The drawing under review shows one solid part. Ordinate dimensions are in mm from its lowest x, y, z. Coordinates: 2 decimals unless noted, no trailing zeros. Loops run counter-clockwise (first coordinate to the right, second up) from the corner with the lowest first, then second, coordinate; pieces in that order, holes last. Notation, with made-up numbers: M -22,16 L 33,16 A21 ccw 33,46 Z; hole C -12.5,37 d9. An arc over 180 degrees is marked long. Use one line per item in the form item = value.
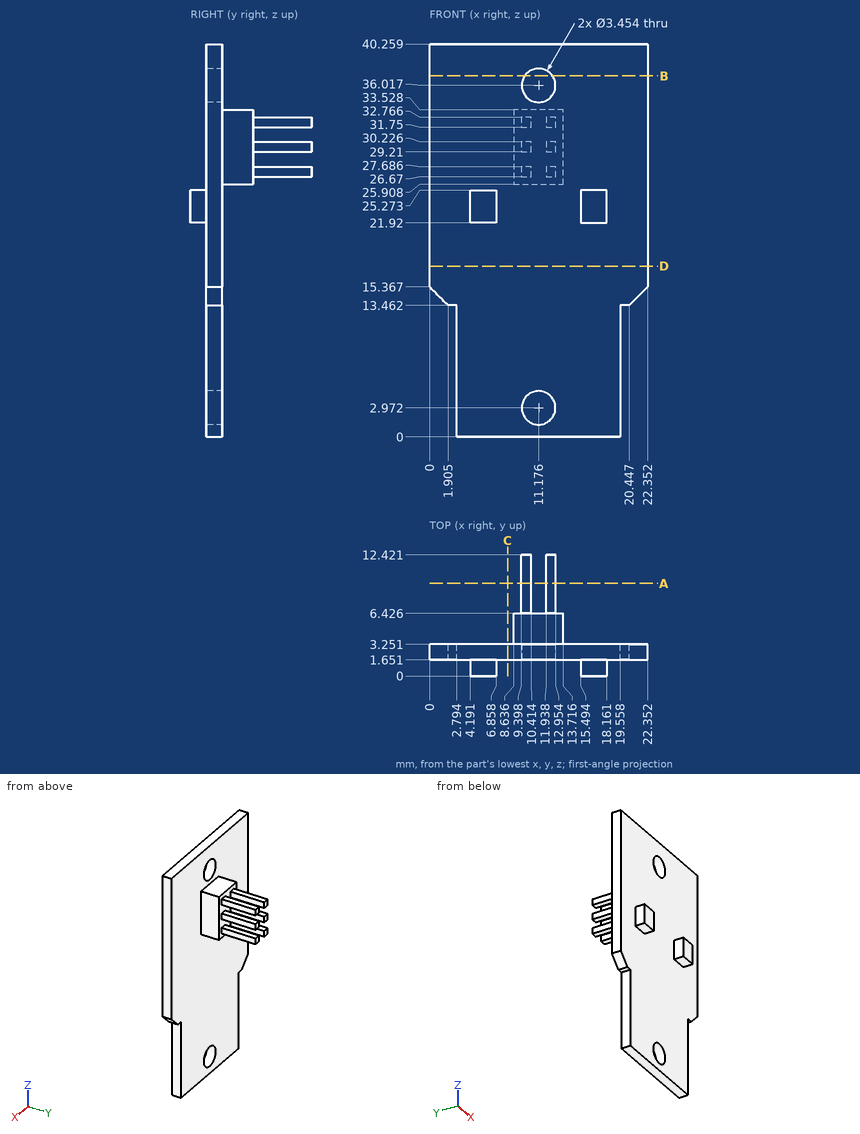
1. Wall thickness on line 1 along Z through (x, y) = (11, 2.5) (1 decimal); line 2 along Y through (x, z) = (6.5, 31.5); line 3 along X through (y, z) = (7.5, 30): over which ranges is each line inside the solid? List them lowest first. Write a range as from..to.
Computed values:
line_1 = 0..1.3, 4.7..34.3, 37.7..40.3
line_2 = 1.65..3.25
line_3 = 9.4..10.41, 11.94..12.95
2. Consider section D-D on z = 17.5. Write out the cut boundary in (x, y).
Computed values:
outline = M 0,1.65 L 22.35,1.65 L 22.35,3.25 L 0,3.25 Z
3. For pin 1 Ø3 at (x, z) = (11.18, 36.02) entering from -Y; pin 2 Ø10 at (x, z) = (2.5, 31.5) entering from +Y; pin 3 Ø0.5 at (x, y) = (6, 1) entering from +Z; pin 4 Ø0.5 at (y, z) = (8.5, 30) entering from +X, all flat-tipped, find the tip position at first contact; note any pin that passes through.
Computed values:
pin_1 = through
pin_2 = 3.25
pin_3 = 25.27
pin_4 = 12.95
4. Consider section C-C on x = 8. Write out the cut boundary in (y, z).
Computed values:
outline = M 1.65,0 L 3.25,0 L 3.25,40.26 L 1.65,40.26 Z
5. Consider section B-B on z = 37. Write out the cut boundary in (x, y) (1 decimal).
Computed values:
outline = M 0,1.7 L 9.8,1.7 L 9.8,3.3 L 0,3.3 Z; M 12.6,1.7 L 22.4,1.7 L 22.4,3.3 L 12.6,3.3 Z
6. Consider section A-A on y = 9.5. Write out the cut boundary in (x, z).
Computed values:
outline = M 9.4,26.67 L 10.41,26.67 L 10.41,27.69 L 9.4,27.69 Z; M 9.4,29.21 L 10.41,29.21 L 10.41,30.23 L 9.4,30.23 Z; M 9.4,31.75 L 10.41,31.75 L 10.41,32.77 L 9.4,32.77 Z; M 11.94,26.67 L 12.95,26.67 L 12.95,27.69 L 11.94,27.69 Z; M 11.94,29.21 L 12.95,29.21 L 12.95,30.23 L 11.94,30.23 Z; M 11.94,31.75 L 12.95,31.75 L 12.95,32.77 L 11.94,32.77 Z
